CAD build for the part. Positions are in the model's coordinates, mm. Face numbers are marked on the shaded views. A direction names the side the tool comes from. Give positions to 0.01 mm unless a question says otherwise; leave off trailing zeros. Order: outer loops, then holes, each group sorted by start corner. A loop starts at its lowest first (then second) coordinate and runs counter-clockwise, first axis right, second up.
from build123d import *

# Parameters (mm, degrees)
F0_W            = 50
F0_H            = 50
F1_DEPTH        = 5
F2_W            = 45
F2_H            = 5
F3_DEPTH        = 45
F4_W            = 36.8
F4_H            = 5
F5_DEPTH        = 45
F6_R            = 25
F7_R            = 2
F10_D           = 3.1
F10_DEPTH       = 20
F10_TIP         = 0.9313339595
F10_ON_F9_D     = 3.1
F10_ON_F9_DEPTH = 20
F10_ON_F9_TIP   = 0.9313339595


with BuildPart() as f1:
    # F0 (on Top) → F1 (new body)
    with BuildSketch(Plane.XY):
        Rectangle(F0_W, F0_H)
    extrude(amount=F1_DEPTH)

    # F2 (on face) → F3 (join)
    with BuildSketch(Plane.XY.offset(5)):
        Polygon((-20, 25), (-25, 25), (-25, -25), (-20, -25), (-20, 20), align=None)
        with Locations((2.5, 22.5)):
            Rectangle(F2_W, F2_H)
    extrude(amount=F3_DEPTH)

    # F4 (on face) → F5 (join, through all)
    with BuildSketch(Plane.XY.offset(5)):
        Polygon((-16.8, 16.8), (-16.8, -25), (-11.8, -25), (-11.8, 11.8), (-11.8, 16.8), align=None)
        with Locations((6.6, 14.3)):
            Rectangle(F4_W, F4_H)
    extrude(amount=F5_DEPTH)

    # F6
    f6_edges = [f1.edges().sort_by_distance(p)[0] for p in [
        (-22.5, -25, 50),
        (-14.3, -25, 50),
        (25, 14.3, 50),
        (25, 22.5, 50),
    ]]
    fillet(f6_edges, radius=F6_R)

    # F7
    f7_edges = [f1.edges().sort_by_distance(p)[0] for p in [
        (25, 25, 12.5),
        (17.67767, 25, 42.67767),
        (0, 25, 0),
        (-12.5, 25, 50),
        (-25, 25, 25),
        (0, -25, 0),
        (25, 0, 0),
        (-25, 0, 0),
        (-25, 12.5, 50),
        (-25, -17.67767, 42.67767),
        (-25, -25, 12.5),
        (-11.8, -6.6, 5),
        (6.6, 11.8, 5),
        (25, -6.6, 5),
        (6.6, -25, 5),
        (-11.8, 11.8, 27.5),
        (-11.8, -25, 15),
        (25, 11.8, 15),
        (-11.8, -17.67767, 42.67767),
        (-11.8, 5.9, 50),
        (17.67767, 11.8, 42.67767),
        (-5.9, 11.8, 50),
    ]]
    fillet(f7_edges, radius=F7_R)

    # F10
    with Locations(Plane.YZ.offset(-11.8)):
        with Locations((-6.6, 27.5)):
            Hole(F10_D / 2, depth=F10_DEPTH)
            with Locations((0, 0, -(F10_DEPTH + F10_TIP / 2))):  # 118° drill point
                Cone(0, F10_D / 2, F10_TIP, mode=Mode.SUBTRACT)

    # F10 on F9
    with Locations(Plane.XZ.offset(-11.8)):
        with Locations((6.6, 27.5)):
            Hole(F10_ON_F9_D / 2, depth=F10_ON_F9_DEPTH)
            with Locations((0, 0, -(F10_ON_F9_DEPTH + F10_ON_F9_TIP / 2))):  # 118° drill point
                Cone(0, F10_ON_F9_D / 2, F10_ON_F9_TIP, mode=Mode.SUBTRACT)


solid = f1.part
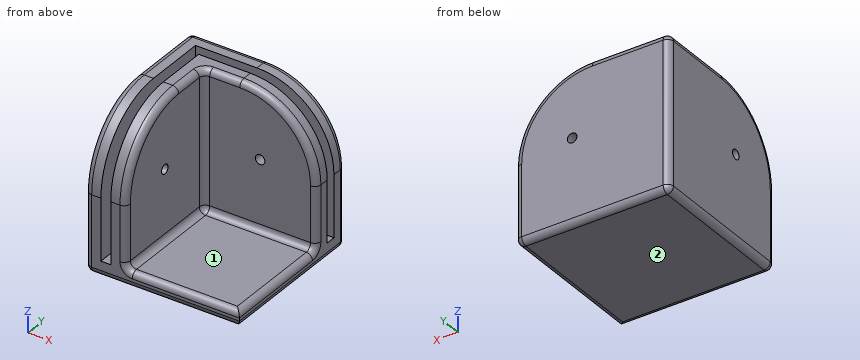
1. Saw through at D-D on y = -6.6. State how many separate pieces and enclosed holes the cut face has, plus the area to 3 significant figures.
2. Wall check: line 1 (X direction, y = 7.5, z = 26.5); line 2 (Y direction, x = 20, z = 28); line 3 (X direction, y = 14, z = 27). Give the ranges that are in metal, low to high.
3. Saw through at B-B on y = 4. Give the cut face in (x, z).
4. Pin check, flat tips, straight feed: P1, Ø4, axis at y = -6.6, z = 27.5, coming from the +X side; P2, Ø12, axis at x = -3, y = 7.5, coming from the +Z side; P3, Ø3, axis at x = 6.6, z = 27.5, coming from the -Y side; P4, Ø2, axis at x = -16.5, y = -14, coming from the +Z side. Stop position of each tip, or through.
5. 3-axis set-ups, long thin cutter, end or side, ignore diameter. For the marked faces 1 and 2: which of +Z, -Z, +X, -X, +Y, -Y reach the whole face in a straight line?
6. Saw through at A-A on z = 22. Give the cut face in (x, y).
7. Saw through at C-C on x = -8. Give the cut face in (y, z), plus the area to 3 significant figures.
Reported:
1. separate pieces: 3
1. enclosed holes: 0
1. area: 657 mm2
2. line 1: x = -25 to -20, -16.8 to -11.8
2. line 2: y = 11.8 to 16.8, 20 to 25
2. line 3: x = -25 to -20, -16.8 to 5.13, 8.07 to 24.92
3. outline: (-25, 2) arc R2 ccw to (-23, 0) - (23, 0) arc R2 ccw to (25, 2) - (25, 3) arc R2 ccw to (23, 5) - (-9.8, 5) arc R2 cw to (-11.8, 7) - (-11.8, 48) arc R2 ccw to (-13.8, 50) - (-16.8, 50) - (-16.8, 5) - (-20, 5) - (-20, 50) - (-23, 50) arc R2 ccw to (-25, 48) - close
4. P1: stops at x = -11.8
4. P2: stops at z = 49.98
4. P3: passes through
4. P4: stops at z = 46.35
5. face 1: +Z, +X, -Y
5. face 2: -Z, +X, -X, +Y, -Y
6. outline: (-25, -23) arc R2 ccw to (-23, -25) - (-20, -25) - (-20, 20) - (25, 20) - (25, 23) arc R2 ccw to (23, 25) - (-23, 25) arc R2 ccw to (-25, 23) - close; (-16.8, -25) - (-13.8, -25) arc R2 ccw to (-11.8, -23) - (-11.8, 9.8) arc R2 cw to (-9.8, 11.8) - (23, 11.8) arc R2 ccw to (25, 13.8) - (25, 16.8) - (-16.8, 16.8) - close
7. outline: (-25, 2) arc R2 ccw to (-23, 0) - (23, 0) arc R2 ccw to (25, 2) - (25, 48) arc R2 ccw to (23, 50) - (20, 50) - (20, 5) - (16.8, 5) - (16.8, 50) - (13.8, 50) arc R2 ccw to (11.8, 48) - (11.8, 7) arc R2 cw to (9.8, 5) - (-23, 5) arc R2 ccw to (-25, 3) - close
7. area: 697 mm2
